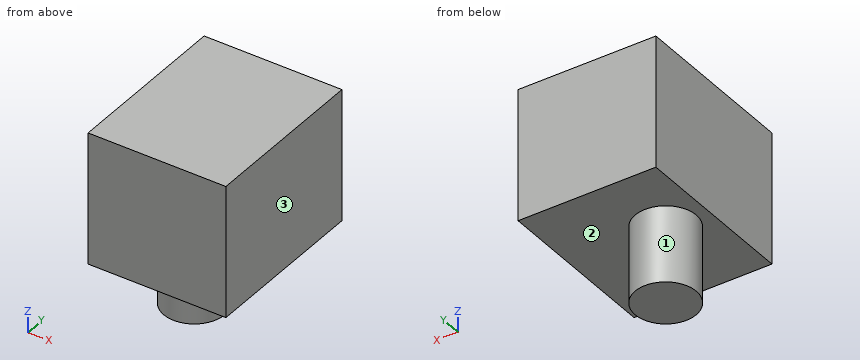
from build123d import *

# Parameters (mm, degrees)
F0_W     = 66.141769
F0_H     = 51.272144
F1_DEPTH = 53.594
F2_R     = 11.874226
F3_DEPTH = 81.026


with BuildPart() as f1:
    # F0 (on Right) → F1 (new body)
    with BuildSketch(Plane.YZ):
        with Locations((-33.070884, 31.703164)):
            Rectangle(F0_W, F0_H)
    extrude(amount=F1_DEPTH)

    # F2 (on face) → F3 (join)
    with BuildSketch(Plane.XY.offset(57.339236)):
        with Locations((16.360093, -29.572813)):
            Circle(F2_R)
    extrude(amount=-F3_DEPTH)


solid = f1.part
Geometry check sheet. Reference: the model listing, model coordinates, mm. Face numbers are marked on the shaded views. Round coordinates to 2 decimals unless told otherwise and drop trailing zeros. Loops run counter-clockwise (first coordinate to the right, second up) from the corner with the lowest first, then second, coordinate; pieces in that order, holes last. Notation, with made-up numbers: (-20.5, 49.25) - (11.5, 49.25) arc R10 cw to (11.5, 59.25) - close; hole circle Ø10 at (-0.75, -37.5). An arc over 180 degrees is marked (long way). One line per question, with ' | ' between items. Start each with the question number.
1. Cross-section at D-D on z = -6. Record the cut outline in (x, y), then the cut area to 3 significant figures.
2. Cross-section at B-B on x = 13. Record the cut outline in (y, z), then the cut area to 3 significant figures.
3. Cross-section at A-A on y = -8.5. Record the cut outline in (x, z), then the cut area to 3 significant figures.
4. Cross-section at C-C on x = 7. Record the cut outline in (y, z).
5. Depth check by flat-ended pin: pin 1 (16 mm diameter, centred on x = 34, y = -46.5, fed in from -Z). Enter the tip coordinate at first touch or a pass-through.
6. Scan lines: line 1 (Z direction, x = 5.5, y = -22.5); line 2 (Y direction, x = 15, z = -7). Record each from-to range of solid material in increasing order. Write a range as [from, to].
7. Draft check along X on the marked faces 1, 2 and 3. Enter one of: released by +X, released by -X, zero draft, split by the parting line, or undercut.
Taken from the geometry:
1) outline: circle Ø23.75 at (16.36, -29.57) | area: 443 mm²
2) outline: (-66.14, 6.07) - (-40.96, 6.07) - (-40.96, -23.69) - (-18.18, -23.69) - (-18.18, 6.07) - (0, 6.07) - (0, 57.34) - (-66.14, 57.34) - close | area: 4,070 mm²
3) outline: (0, 6.07) - (53.59, 6.07) - (53.59, 57.34) - (0, 57.34) - close | area: 2,750 mm²
4) outline: (-66.14, 6.07) - (-36.88, 6.07) - (-36.88, -23.69) - (-22.27, -23.69) - (-22.27, 6.07) - (0, 6.07) - (0, 57.34) - (-66.14, 57.34) - close
5) pin 1: z = 6.07
6) line 1: [6.07, 57.34] | line 2: [-41.37, -17.78]
7) face 1: split by the parting line | face 2: zero draft | face 3: released by +X
